```python
from build123d import *

# Parameters (mm, degrees)
CHAFL_N1_SIZE         = 2
CORTAR_EXTRUIR1_DEPTH = 10


with BuildPart() as part:
    # Croquis1 → Revolución1 (revolve)
    with BuildSketch(Plane.XY):
        Polygon((0, 0), (0, 27.5), (177, 27.5), (177, 32.725), (242, 32.725), (242, 27.5), (432, 27.5), (432, 0), align=None)
    revolve(axis=Axis((432, 0, 0), (-1, 0, 0)))

    # Chaflán1
    chafl_n1_edges = [part.edges().sort_by_distance(p)[0] for p in [
        (432, -27.5, 0),
        (0, -27.5, 0),
    ]]
    chamfer(chafl_n1_edges, length=CHAFL_N1_SIZE)

    # Croquis2 → Cortar-Extruir1 (cut)
    with BuildSketch(Plane(origin=(0, 27.5, 0), x_dir=(1, 0, 0), z_dir=(0, 1, 0))):
        with BuildLine():
            Line((57, 5), (12, 5))
            ThreePointArc((12, 5), (7, 0), (12, -5))
            Line((12, -5), (57, -5))
            ThreePointArc((57, -5), (62, 0), (57, 5))
        make_face()
    extrude(amount=-CORTAR_EXTRUIR1_DEPTH, mode=Mode.SUBTRACT)


solid = part.part
```
Geometry check sheet. Reference: the model listing, model coordinates, mm. A direction names the side the tool comes from. Coordinates: 2 decimals unless noted, no trailing zeros. Order: outer loops, then holes, each group sorted by start corner. A loop starts at its lowest first (then second) coordinate and runs counter-clockwise, first axis right, second up. Notation, with made-up numbers: M -19,39.5 L -11,39.5 A10 ccw -11,53.5 Z; hole C 14.25,45 d6. An arc over 180 degrees is marked long. Answer as a JSON object with one key per item and string values.
Q1. Tool access check on faces 1 (the flat face through (34, 22, 5)), 2 (the cylindrical face through (337.316, -5.961, 26.846)), 3 (the cylindrical face through (90.725, -5.961, 26.846)). Record the directions out of +Z, -Z, +X, -X, +Y, -Y that give a thin tool (end or side, any length) a straight path to the whole face; none if there is none.
Results are:
{"face 1": "+Y", "face 2": "+X", "face 3": "-X"}
Q2. Cross-section at B-B on x = 355. Record the cut outline in (y, z), and give its area (3 significant figures).
Results are:
{"outline": "C 0,0 d55", "area": "2,380 mm²"}
Q3. Cross-section at A-A on z = 0. Record the cut outline in (x, y) (3 decimals).
Results are:
{"outline": "M 0,-25.5 L 2,-27.5 L 177,-27.5 L 177,-32.725 L 242,-32.725 L 242,-27.5 L 430,-27.5 L 432,-25.5 L 432,25.5 L 430,27.5 L 242,27.5 L 242,32.725 L 177,32.725 L 177,27.5 L 62,27.5 L 62,17.5 L 7,17.5 L 7,27.5 L 2,27.5 L 0,25.5 Z"}
Q4. Cross-section at C-C on x = 196. Record the cut outline in (y, z) (3 decimals).
Results are:
{"outline": "C 0,0 d65.45"}
Q5. Release check for a two-part mould opening along X. For faces 4 (the flat face through (35, 22, -5)), 5 (the conical face through (0.125, 24.442, -7.697)), 6 (the flat face through (242, -7, -27)) record: released by +X, released by -X, zero draft, split by the parting line, or undercut.
Results are:
{"face 4": "undercut", "face 5": "released by -X", "face 6": "released by +X"}
Q6. Scan lines: line 1 (X direction, y = 4, z = -27.5); line 2 (Z direction, x = 214, y = 26); line 3 (Z direction, x = 56.5, y = -10.5). Record each from-to range of solid material in increasing order.
Results are:
{"line 1": "x = 177 to 242", "line 2": "z = -19.87 to 19.87", "line 3": "z = -25.42 to 25.42"}
Q7. Depth check by flat-ended pin: pin 1 Ø5 at (x, y) = (37.5, 21) entering from -Z; pin 2 Ø2 at (y, z) = (26, 3) entering from -X; pin 3 Ø11 at (x, z) = (29.5, -1.5) entering from +Y; pin 4 Ø2 at (x, y) = (373.5, -23) entering from +Z. Enter the tip coordinate at first touch or a pass-through.
Results are:
{"pin 1": "stops at z = -20.35", "pin 2": "stops at x = 0", "pin 3": "stops at y = 27.04", "pin 4": "stops at z = 16.5"}
